from build123d import *

# Parameters (mm, degrees)
SKETCH040_W             = 40.7
SKETCH040_H             = 20.15
PAD020_DEPTH            = 29
PAD021_DEPTH            = 2.55
SKETCH042_W             = 40.7
SKETCH042_H             = 20.15
PAD022_DEPTH            = 5.5
PAD023_DEPTH            = 2
SKETCH044_R             = 6.5
PAD024_DEPTH            = 1.3
SKETCH045_R             = 5.5
PAD025_DEPTH            = 0.7
SKETCH046_R             = 3
PAD026_DEPTH            = 3.5
BODY013_PLACEMENT_ANGLE = 180
BODY046_PLACEMENT_ANGLE = 180


with BuildPart() as part:
    # Sketch040 → Pad020 (new body)
    with BuildSketch(Plane.XY):
        Rectangle(SKETCH040_W, SKETCH040_H)
    extrude(amount=-PAD020_DEPTH)

    # Sketch041 (on Face5 of Pad020) → Pad021 (join)
    with BuildSketch(Plane.XY):
        with BuildLine():
            Line((-27.2, 10.075), (27.2, 10.075))
            Line((27.2, 10.075), (27.2, 6))
            ThreePointArc((27.2, 6), (21.620764, 5), (27.2, 4))
            Line((27.2, 4), (27.2, -4))
            ThreePointArc((27.2, -4), (21.620764, -5), (27.2, -6))
            Line((27.2, -6), (27.2, -10.075))
            Line((27.2, -10.075), (-27.2, -10.075))
            Line((-27.2, -10.075), (-27.2, -6))
            ThreePointArc((-27.2, -6), (-21.620764, -5), (-27.2, -4))
            Line((-27.2, 4), (-27.2, -4))
            ThreePointArc((-27.2, 4), (-21.620764, 5), (-27.2, 6))
            Line((-27.2, 10.075), (-27.2, 6))
        make_face()
    extrude(amount=PAD021_DEPTH)

    # Sketch042 (on Face5 of Pad021) → Pad022 (join)
    with BuildSketch(Plane.XY.offset(2.55)):
        Rectangle(SKETCH042_W, SKETCH042_H)
    extrude(amount=PAD022_DEPTH)

    # Sketch043 (on Face21 of Pad022) → Pad023 (join)
    with BuildSketch(Plane.XY.offset(8.05)):
        with BuildLine():
            ThreePointArc((5.991101, -9), (20.35, 0), (5.991101, 9))
            Line((5.991101, 9), (-14.85, 9))
            Line((-14.85, 9), (-14.85, 5))
            ThreePointArc((-14.85, 5), (-16.69017, 2.795085), (-17.35, 0))
            ThreePointArc((-17.35, 0), (-16.69017, -2.795085), (-14.85, -5))
            Line((-14.85, -5), (-14.85, -9))
            Line((-14.85, -9), (5.991101, -9))
        make_face()
    extrude(amount=PAD023_DEPTH)

    # Sketch044 (on Face34 of Pad023) → Pad024 (join)
    with BuildSketch(Plane.XY.offset(10.05)):
        with Locations((10.35, 0)):
            Circle(SKETCH044_R)
    extrude(amount=PAD024_DEPTH)

    # Sketch045 (on Face36 of Pad024) → Pad025 (join)
    with BuildSketch(Plane.XY.offset(11.35)):
        with Locations((10.35, 0)):
            Circle(SKETCH045_R)
    extrude(amount=PAD025_DEPTH)

    # Sketch046 (on Face38 of Pad025) → Pad026 (join)
    with BuildSketch(Plane.XY.offset(12.05)):
        with Locations((10.35, 0)):
            Circle(SKETCH046_R)
    extrude(amount=PAD026_DEPTH)


with BuildPart() as part_1:
    # Body013 placement: moved
    add(part.part.moved(Location((-58.5, 0, 88.5))).rotate(Axis((-58.5, 0, 88.5), (1, 0, 0)), BODY013_PLACEMENT_ANGLE))


with BuildPart() as part_2:
    # Body046 placement: moved
    add(part_1.part.rotate(Axis((0, 0, 0), (0, 0, 1)), BODY046_PLACEMENT_ANGLE))


solid = part_2.part
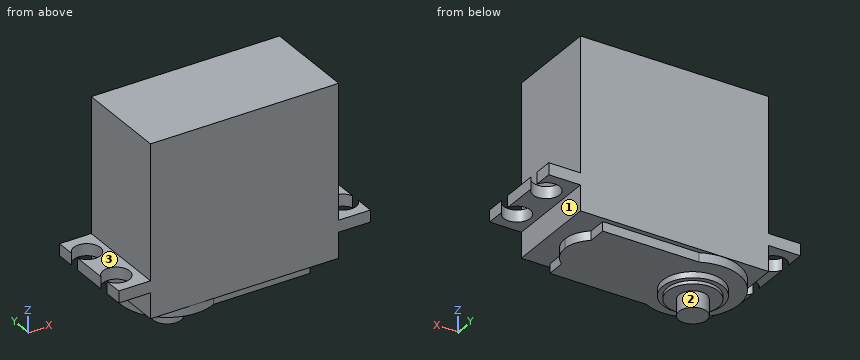
Geometry: final body of the model. Coordinates: model frame, mm. Face numbers are marked on the shaded views. A direction names the side the tool comes from. Coordinates: 2 decimals unless noted, no trailing zeros. Order: outer loops, then holes, each group sorted by start corner. A loop starts at its lowest first (then second) coordinate and runs counter-clockwise, first axis right, second up.
1) Set-up query: the marked faces 1, 2 and 3. Return all of +Z, -Z, +X, -X, +Y, -Y with unobstructed straight access to the full face (end or side cutting, diameter ignored); none if empty.
Result sheet:
face 1: -Z, +X, +Y, -Y
face 2: -Z
face 3: +Z, -X, +Y, -Y
2) Section A-A (x = 34). Return loops of the section in (y, z) (3 decimals), then the cut area to 3 significant figures.
Result sheet:
outline: (-10.075, 85.95) - (-7.879, 85.95) - (-7.879, 88.5) - (-10.075, 88.5) - close; (-2.121, 85.95) - (2.121, 85.95) - (2.121, 88.5) - (-2.121, 88.5) - close; (7.879, 85.95) - (10.075, 85.95) - (10.075, 88.5) - (7.879, 88.5) - close
area: 22.0 mm2
3) Ray query, probe 1 along Y at (x, z) = (34, 86.6) (3 decimals); probe 2 along Z at (x, y) = (49, 6.75); probe 3 along Z at (x, y) = (52.5, -1). Return the intervals inside material, ascending.
Result sheet:
probe 1: y = -10.075 to -7.879, -2.121 to 2.121, 7.879 to 10.075
probe 2: z = 78.45 to 117.5
probe 3: z = 76.45 to 117.5
4) First-contact query: P1, Ø4, axis at x = 50, y = 6.5, coming from the -Z side; P2, Ø6, axis at x = 65.5, y = 1, coming from the -Z side; P3, Ø7.5, axis at x = 83, y = 5, coming from the -Z side; P4, Ø1, axis at y = 8, z = 77.5, coming from the +X side. Flat tips, straight axial feed; report the tip coordinate or a pass-through.
Result sheet:
P1: stops at z = 76.45
P2: stops at z = 78.45
P3: stops at z = 85.95
P4: passes through
5) Section B-B (x = 63.5). Return loops of the section in (y, z) (3 decimals).
Result sheet:
outline: (-10.075, 80.45) - (-9, 80.45) - (-9, 78.45) - (9, 78.45) - (9, 80.45) - (10.075, 80.45) - (10.075, 117.5) - (-10.075, 117.5) - close
6) Section C-C (y = -1.25). Return loops of the section in (x, z), then the cut area to 3 significant figures.
Result sheet:
outline: (31.3, 85.95) - (38.15, 85.95) - (38.15, 80.45) - (38.23, 80.45) - (38.23, 78.45) - (41.77, 78.45) - (41.77, 77.15) - (42.79, 77.15) - (42.79, 76.45) - (45.42, 76.45) - (45.42, 72.95) - (50.88, 72.95) - (50.88, 76.45) - (53.51, 76.45) - (53.51, 77.15) - (54.53, 77.15) - (54.53, 78.45) - (75.72, 78.45) - (75.72, 80.45) - (78.85, 80.45) - (78.85, 85.95) - (85.7, 85.95) - (85.7, 88.5) - (78.85, 88.5) - (78.85, 117.5) - (38.15, 117.5) - (38.15, 88.5) - (31.3, 88.5) - close
area: 1,660 mm2
7) Section D-D (z = 85). Return loops of the section in (x, y) (3 decimals), then the cut area to 3 significant figures.
Result sheet:
outline: (38.15, -10.075) - (78.85, -10.075) - (78.85, 10.075) - (38.15, 10.075) - close
area: 820 mm2
